Part print with two shaded views. Sizes in mm from the minimum x, y, z corner. A direction names the side the tool comes from. Round coordinates to 2 decimals unless told otherwise and drop trailing zeros. Write each loop counter-clockwise with the first axis right and the second up, starting at its lowest first coordinate (ties: lowest second). Pieces come first, ordered by that corner, then holes. Notation, with made-up numbers: (49.5, 35) -> (105.5, 35) arc R35 cw to (105.5, 67) -> close; hole circle Ø1 at (15, 37.25). An arc over 180 degrees is marked (long way). Answer in a Markdown table with one row per item.
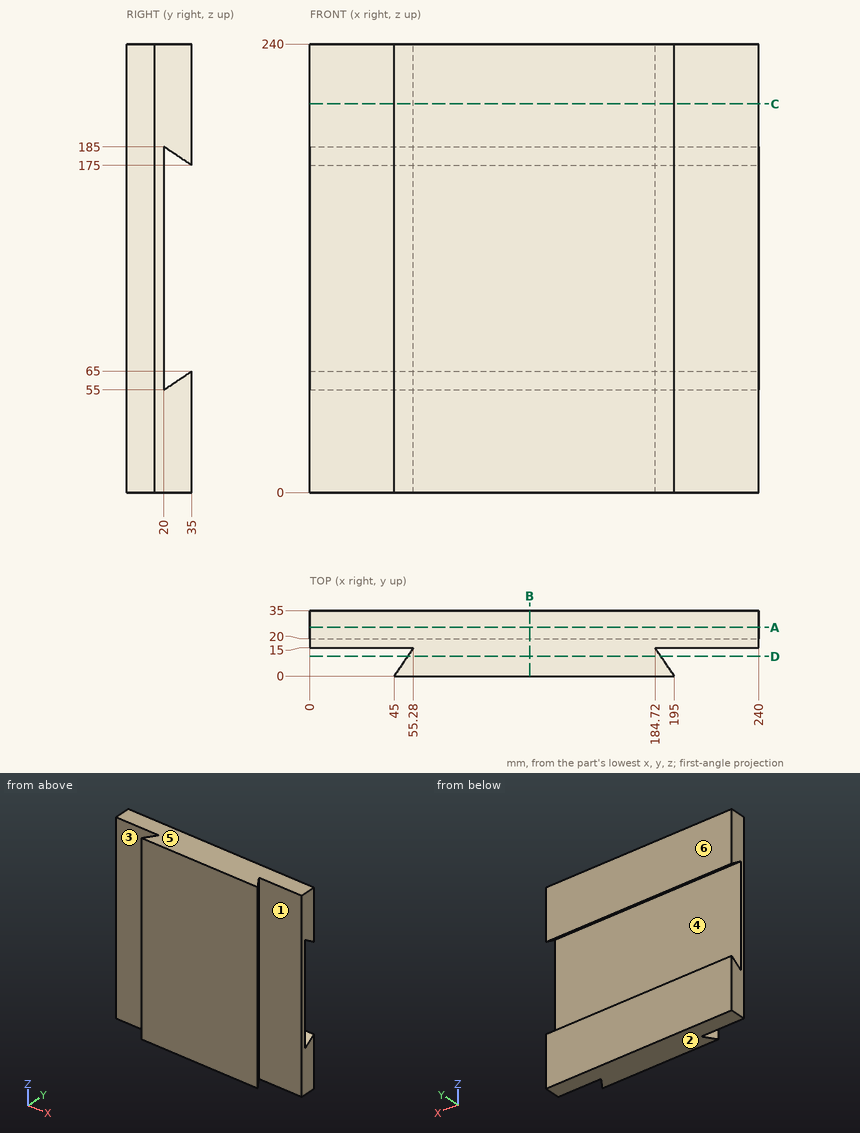
Q1. Which spindle directions (+Z, -Z, +X, -X, +Y, -Y) get a long thin tool onto all of the face, cutting with end or side? Do the marked faces 1, 2 and 3. Say none if no direction does.
A:
| item | result |
|---|---|
| face 1 | +Z, -Z, +X |
| face 2 | -Z, +X, -X, +Y, -Y |
| face 3 | +Z, -Z, -X |
Q2. Wall check: line 1 (Z direction, x = 165.5, y = 25.5); line 2 (Y direction, x = 142.5, z = 130.5); line 3 (Z direction, x = 134, y = 28.5). Give the ranges that are in metal, low to high. Write a range as [from, to].
A:
| item | result |
|---|---|
| line 1 | [0, 58.67], [181.33, 240] |
| line 2 | [0, 20] |
| line 3 | [0, 60.67], [179.33, 240] |
Q3. Saw through at A-A on y = 26. Write the cut outline in (x, z), plus the area to 3 significant figures.
A:
| item | result |
|---|---|
| outline | (0, 0) -> (240, 0) -> (240, 59) -> (0, 59) -> close; (0, 181) -> (240, 181) -> (240, 240) -> (0, 240) -> close |
| area | 28,300 mm² |
Q4. Two-plate mould, pull along Z, no slides. Class the marked faces 4, 5 and 6: released by +Z, released by -Z, zero draft, split by the parting line, or undercut.
A:
| item | result |
|---|---|
| face 4 | undercut |
| face 5 | released by +Z |
| face 6 | zero draft |
Q5. Saw through at D-D on y = 10.5. Write the cut outline in (x, z).
A:
| item | result |
|---|---|
| outline | (52.2, 0) -> (187.8, 0) -> (187.8, 240) -> (52.2, 240) -> close |
Q6. Saw through at B-B on x = 117.5. Write the cut outline in (y, z), plus the area to 3 significant figures.
A:
| item | result |
|---|---|
| outline | (0, 0) -> (35, 0) -> (35, 65) -> (20, 55) -> (20, 185) -> (35, 175) -> (35, 240) -> (0, 240) -> close |
| area | 6,600 mm² |
Q7. Drop a flat-ended pin along its axis: P1, Ø1, axis at x = 208, z = 169, coming from the -Y side. Give the stop position or say it passes through.
A:
| item | result |
|---|---|
| P1 | y = 15 |
Q8. Saw through at C-C on z = 208. Write the cut outline in (x, y), plus the area to 3 significant figures.
A:
| item | result |
|---|---|
| outline | (0, 15) -> (55.28, 15) -> (45, 0) -> (195, 0) -> (184.72, 15) -> (240, 15) -> (240, 35) -> (0, 35) -> close |
| area | 6,900 mm² |
